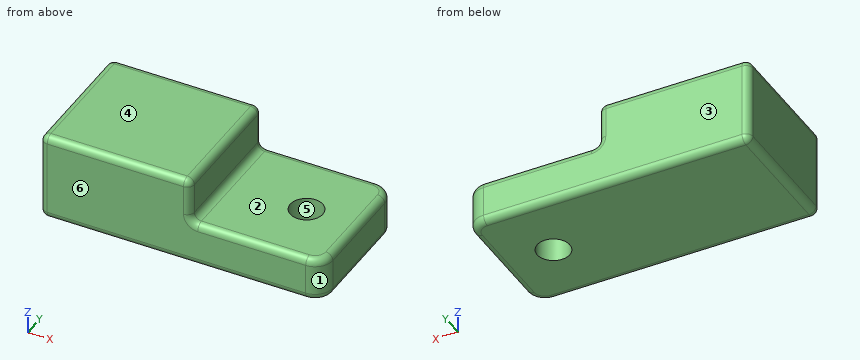
from build123d import *

# Parameters (mm, degrees)
F0_W      = 107.95
F0_H      = 95.25
F1_DEPTH  = 63.5
F0_R      = 11.66987
F2_DEPTH  = 25.4
F2_FACE_R = 11.66987
F3_DEPTH  = 6.35
F4_R      = 5.08


with BuildPart() as f1:
    # F0 (on Top) → F1 (new body)
    with BuildSketch(Plane.XY):
        with Locations((-149.225, 47.625)):
            Rectangle(F0_W, F0_H)
    extrude(amount=F1_DEPTH)

    # F0 (on Top) → F2 (join)
    with BuildSketch(Plane.XY):
        with BuildLine():
            Line((-12.7, 95.25), (-95.25, 95.25))
            Line((-95.25, 95.25), (-95.25, 0))
            Line((-95.25, 0), (-12.7, 0))
            ThreePointArc((-12.7, 0), (-3.719744, 3.719744), (0, 12.7))
            Line((0, 12.7), (0, 82.55))
            ThreePointArc((0, 82.55), (-3.719744, 91.530256), (-12.7, 95.25))
        make_face()
        with Locations((-37.450853, 47.625)):
            Circle(F0_R, mode=Mode.SUBTRACT)
    extrude(amount=F2_DEPTH)

    # F2_face (on face) → F3 (join)
    with BuildSketch(Plane(origin=(-48.494155, 47.625, 25.4), x_dir=(1, 0, 0), z_dir=(0, 0, 1))):
        with BuildLine():
            Line((35.794155, 47.625), (-46.755845, 47.625))
            Line((-46.755845, 47.625), (-46.755845, -47.625))
            Line((-46.755845, -47.625), (35.794155, -47.625))
            ThreePointArc((35.794155, -47.625), (44.774411, -43.905256), (48.494155, -34.925))
            Line((48.494155, -34.925), (48.494155, 34.925))
            ThreePointArc((48.494155, 34.925), (44.774411, 43.905256), (35.794155, 47.625))
        make_face()
        with Locations((11.043302, 0)):
            Circle(F2_FACE_R, mode=Mode.SUBTRACT)
    extrude(amount=F3_DEPTH)

    # F4
    f4_edges = [f1.edges().sort_by_distance(p)[0] for p in [
        (0, 12.7, 15.875),
        (0, 47.625, 31.75),
        (0, 82.55, 15.875),
        (0, 47.625, 0),
        (-95.25, 95.25, 47.625),
        (-95.25, 47.625, 63.5),
        (-95.25, 0, 47.625),
        (-95.25, 47.625, 31.75),
        (-149.225, 95.25, 63.5),
        (-203.2, 47.625, 63.5),
        (-149.225, 0, 63.5),
        (-203.2, 95.25, 31.75),
        (-203.2, 0, 31.75),
        (-203.2, 47.625, 0),
    ]]
    fillet(f4_edges, radius=F4_R)


solid = f1.part
Model file for the job. Use its own axes, mm. Face numbers are marked on the shaded views. A direction names the side the tool comes from. Give positions to 0.01 mm unless a question says otherwise; leave off trailing zeros. Order: outer loops, then holes, each group sorted by start corner. A loop starts at its lowest first (then second) coordinate and runs counter-clockwise, first axis right, second up. Notation, with made-up numbers: M 31.5,-1.5 L 80.5,-1.5 A21 cw 80.5,26.5 Z; hole C -36,-7 d9. An arc over 180 degrees is marked long. Put each result on its own line as item: value. Start each with the question number.
(1) Band-saw the part on B-B on y = 42.5. Give the cut face in (x, z), then the cut area to 3 significant figures.
(2) Drill centre lines: L1, parallel to X at y = 14, z = 40.5; L2, parallel to Z at x = -72, y = 50; L3, parallel to X at y = 58, z = 21.5. Where is each one in solid material? Low to high. Write a range as [from, to].
(3) Band-saw the part on A-A on x = -35.5. Give the cut face in (y, z).
(4) Band-saw the part on D-D on x = -15. Give the cut face in (y, z).
(5) Band-saw the part on C-C on z = 40.5. Give the cut face in (x, y), then the cut area to 3 significant figures.
(6) Pin check, flat tip, straight feed: pin 1 Ø6.5 at (y, z) = (33, 49) entering from +X. Stop position of the tip, or through.
(7) Pull direction Y, two halves, no side cores. Call the marked faces 3, 4, 5 and 6: released by +Y, released by -Y, zero draft, split by the parting line, or undercut.
(8) Tool access for the marked faces 1 and 2: list every direction of +Z, -Z, +X, -X, +Y, -Y with a clear straight run to the whole face (end or side of a thin tool).
Results below:
1. outline: M -203.2,5.08 A5.08 ccw -198.12,0 L -47.94,0 L -47.94,31.75 L -90.17,31.75 A5.08 cw -95.25,36.83 L -95.25,58.42 A5.08 ccw -100.33,63.5 L -198.12,63.5 A5.08 ccw -203.2,58.42 Z; M -26.97,0 L -5.08,0 A5.08 ccw 0,5.08 L 0,26.67 A5.08 ccw -5.08,31.75 L -26.97,31.75 Z
1. area: 9,190 mm2
2. L1: x = [-203.2, -95.25]
2. L2: z = [0, 31.75]
2. L3: x = [-203.2, -42.79], [-32.11, 0]
3. outline: M 0,5.08 A5.08 ccw 5.08,0 L 36.12,0 L 36.12,31.75 L 5.08,31.75 A5.08 ccw 0,26.67 Z; M 59.13,0 L 90.17,0 A5.08 ccw 95.25,5.08 L 95.25,26.67 A5.08 ccw 90.17,31.75 L 59.13,31.75 Z
4. outline: M 0,5.08 A5.08 ccw 5.08,0 L 90.17,0 A5.08 ccw 95.25,5.08 L 95.25,26.67 A5.08 ccw 90.17,31.75 L 5.08,31.75 A5.08 ccw 0,26.67 Z
5. outline: M -203.2,5.08 A5.08 ccw -198.12,0 L -100.33,0 A5.08 ccw -95.25,5.08 L -95.25,90.17 A5.08 ccw -100.33,95.25 L -198.12,95.25 A5.08 ccw -203.2,90.17 Z
5. area: 10,300 mm2
6. pin 1: stops at x = -95.25
7. face 3: released by +Y
7. face 4: zero draft
7. face 5: undercut
7. face 6: released by -Y
8. face 1: +Z, -Z, +X, -Y
8. face 2: +Z, +X, +Y, -Y
